```python
from build123d import *

# Parameters (mm, degrees)
SKETCH1_R           = 1.3
BOSS_EXTRUDE1_DEPTH = 2.6
SKETCH2_R           = 3
CUT_EXTRUDE1_DEPTH  = 2
CHAMFER1_SIZE       = 0.4
CHAMFER1_SIZE2      = 2.268512728
CHAMFER2_SIZE       = 0.5
CHAMFER2_SIZE2      = 1.866025404
CHAMFER3_SIZE       = 0.3
CHAMFER3_SIZE2      = 0.519615242


with BuildPart() as part:
    # Sketch1 → Boss-Extrude1 (new body)
    with BuildSketch(Plane.XY):
        with BuildLine():
            Line((-8.048780488, 2.43902439), (-2.195121951, 3.756097561))
            ThreePointArc((-2.195121951, 3.756097561), (0, 4), (2.195121951, 3.756097561))
            Line((2.195121951, 3.756097561), (8.048780488, 2.43902439))
            ThreePointArc((8.048780488, 2.43902439), (10, 0), (8.048780488, -2.43902439))
            Line((8.048780488, -2.43902439), (2.195121951, -3.756097561))
            ThreePointArc((2.195121951, -3.756097561), (0, -4), (-2.195121951, -3.756097561))
            Line((-2.195121951, -3.756097561), (-8.048780488, -2.43902439))
            ThreePointArc((-8.048780488, -2.43902439), (-10, 0), (-8.048780488, 2.43902439))
        make_face()
        with Locations((7.5, 0)):
            Circle(SKETCH1_R, mode=Mode.SUBTRACT)
        with Locations((-7.5, 0)):
            Circle(SKETCH1_R, mode=Mode.SUBTRACT)
    extrude(amount=BOSS_EXTRUDE1_DEPTH)

    # Sketch2 → Cut-Extrude1 (cut)
    with BuildSketch(Plane.XY.offset(2.6)):
        Circle(SKETCH2_R)
    extrude(amount=-CUT_EXTRUDE1_DEPTH, mode=Mode.SUBTRACT)

    # Chamfer1
    chamfer1_edges = [part.edges().sort_by_distance(p)[0] for p in [
        (-5.12195122, -3.097560976, 0),
        (-10, 0, 0),
        (-5.12195122, 3.097560976, 0),
        (0, 4, 0),
        (5.12195122, 3.097560976, 0),
        (10, 0, 0),
        (5.12195122, -3.097560976, 0),
        (0, -4, 0),
    ]]
    chamfer1_side = [part.faces().sort_by_distance(p)[0] for p in [
        (0, 0, 0),
    ]]
    chamfer(chamfer1_edges, length=CHAMFER1_SIZE, length2=CHAMFER1_SIZE2, reference=chamfer1_side[0])

    # Chamfer2
    chamfer2_edges = [part.edges().sort_by_distance(p)[0] for p in [
        (-3, 0, 2.6),
    ]]
    chamfer2_side = [part.faces().sort_by_distance(p)[0] for p in [
        (-5.074666846, 2.887408203, 2.6),
    ]]
    chamfer(chamfer2_edges, length=CHAMFER2_SIZE, length2=CHAMFER2_SIZE2, reference=chamfer2_side[0])

    # Chamfer3
    chamfer3_edges = [part.edges().sort_by_distance(p)[0] for p in [
        (6.2, 0, 2.6),
        (-8.8, 0, 2.6),
    ]]
    chamfer3_side = [part.faces().sort_by_distance(p)[0] for p in [
        (-3.715406592, 0, 2.6),
    ]]
    chamfer(chamfer3_edges, length=CHAMFER3_SIZE, length2=CHAMFER3_SIZE2, reference=chamfer3_side[0])


solid = part.part
```
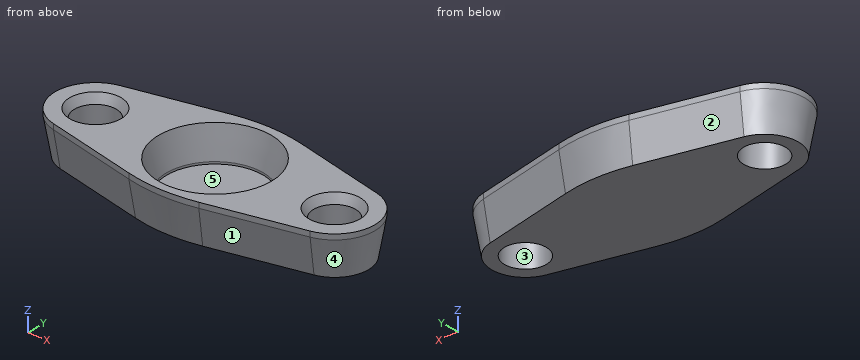
Verification items for the finished model (mm, model axes). Face numbers are marked on the shaded views. A direction names the side the tool comes from. Round coordinates to 2 decimals unless told otherwise and drop trailing zeros. Order: outer loops, then holes, each group sorted by start corner. A loop starts at its lowest first (then second) coordinate and runs counter-clockwise, first axis right, second up. Notation, with made-up numbers: (-37, 25.5) -> (1, 25.5) arc R18 cw to (1, 47.5) -> close; hole circle Ø4 at (-31.75, 59.5). An arc over 180 degrees is marked (long way). Put each result on its own line as item: value. Start each with the question number.
(1) Draft check along Y on the marked faces 1, 2 and 3. Enter one of: +Y half, -Y half, draft (parallel to the pull), parting line (faces both ways), or undercut.
(2) Section check C-C (x = -7.5). Enter the section's corners in (y, z).
(3) Section check A-A (y = 0). Enter the section's corners in (x, z).
(4) Section check D-D (z = 1.15). Enter the section's corners in (x, y).
(5) Material ranges on line 1 along X through (y, z) = (1, 1.7); line 2 along X through (y, z) = (1, 0.2); line 3 along X through (y, z) = (-1, 1.5), recorded low to high.
(6) Section check B-B (z = 0.25). Enter the section's corners in (x, y).
(7) Tool access check on the marked faces 4 and 5. Record the directions out of +Z, -Z, +X, -X, +Y, -Y that give a thin tool (end or side, any length) a straight path to the whole face; none if there is none.
Completed:
1. face 1: -Y half
1. face 2: +Y half
1. face 3: undercut
2. outline: (-2.56, 2.27) -> (-2.15, 0) -> (-1.3, 0) -> (-1.3, 2.08) -> (-1.6, 2.6) -> (-2.56, 2.6) -> close; (1.3, 0) -> (2.15, 0) -> (2.56, 2.27) -> (2.56, 2.6) -> (1.6, 2.6) -> (1.3, 2.08) -> close
3. outline: (-10, 2.27) -> (-9.6, 0) -> (-8.8, 0) -> (-8.8, 2.08) -> (-9.1, 2.6) -> (-10, 2.6) -> close; (-6.2, 0) -> (6.2, 0) -> (6.2, 2.08) -> (5.9, 2.6) -> (3.5, 2.6) -> (3, 0.73) -> (3, 0.6) -> (-3, 0.6) -> (-3, 0.73) -> (-3.5, 2.6) -> (-5.9, 2.6) -> (-6.2, 2.08) -> close; (8.8, 0) -> (9.6, 0) -> (10, 2.27) -> (10, 2.6) -> (9.1, 2.6) -> (8.8, 2.08) -> close
4. outline: (-8.01, -2.25) -> (-2.15, -3.56) arc R9.8 ccw to (2.15, -3.56) -> (8.01, -2.25) arc R2.3 ccw to (8.01, 2.25) -> (2.15, 3.56) arc R9.8 ccw to (-2.15, 3.56) -> (-8.01, 2.25) arc R2.3 ccw to start; hole circle Ø2.6 at (-7.5, 0); hole circle Ø6.22 at (0, 0); hole circle Ø2.6 at (7.5, 0)
5. line 1: x = -9.68 to -8.33, -6.67 to -3.1, 3.1 to 6.67, 8.33 to 9.68
5. line 2: x = -9.39 to -8.33, -6.67 to 6.67, 8.33 to 9.39
5. line 3: x = -9.64 to -8.33, -6.67 to -3.05, 3.05 to 6.67, 8.33 to 9.64
6. outline: (-7.97, -2.09) -> (-2.12, -3.41) arc R9.64 ccw to (2.12, -3.41) -> (7.97, -2.09) arc R2.14 ccw to (7.97, 2.09) -> (2.12, 3.41) arc R9.64 ccw to (-2.12, 3.41) -> (-7.97, 2.09) arc R2.14 ccw to start; hole circle Ø2.6 at (-7.5, 0); hole circle Ø2.6 at (7.5, 0)
7. face 4: -Z, +X
7. face 5: +Z
